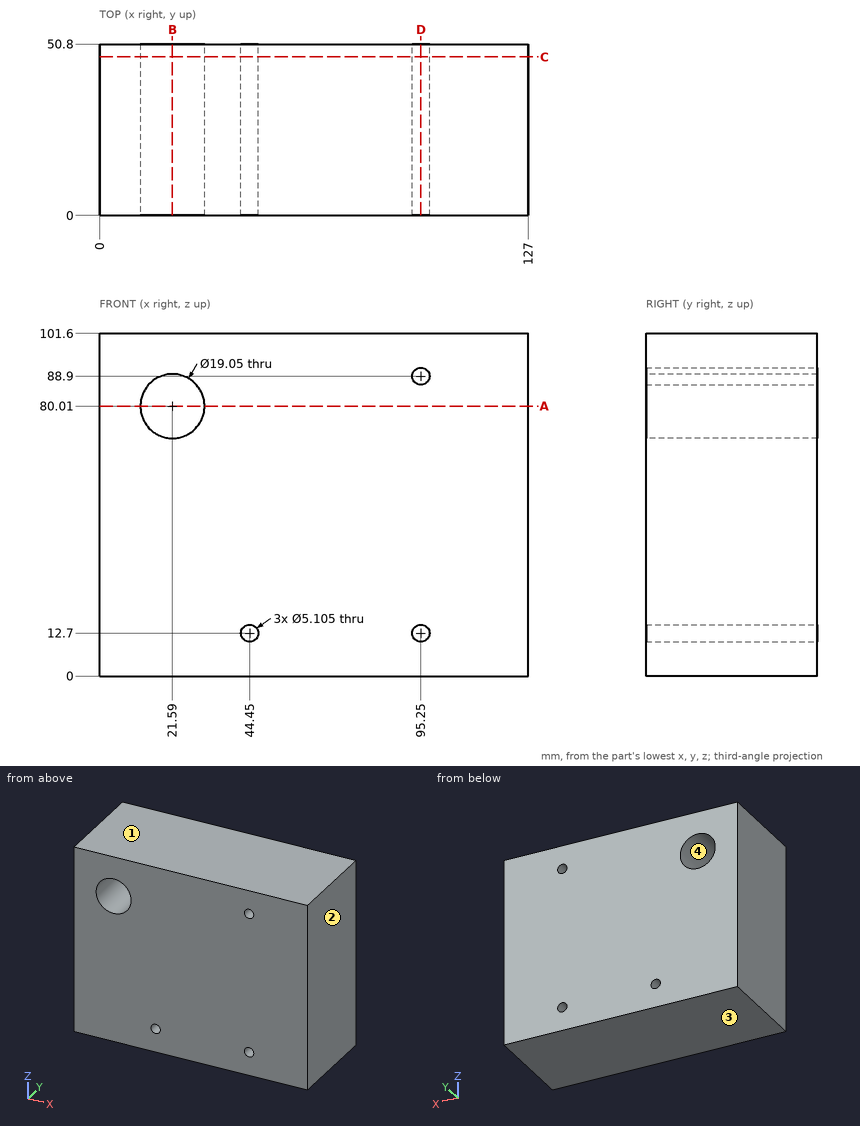
Study the drawing (mm; zero at the part's minimum x, y, z) and answer. Give positions to 0.01 mm unless a question says otherwise; leave off trailing zeros. Loops run counter-clockwise (first coordinate to the right, second up) from the corner with the lowest first, then second, coordinate; pieces in that order, holes last. Notation, with made-up numbers: M 23,79 L 28,79 A25 cw 28,108 Z; hole C 63,68 d6. An arc over 180 degrees is marked long. Answer as CSV lines item,"result".
Item 1: Straight lines are drawn through the part: line 1 along Z through (x, y) = (95.25, 40.5); line 2 along Z through (x, y) = (21.59, 14) (1 decimal); line 3 along X through (y, z) = (29, 80) (1 decimal). For each, find the intervals that lie inside material, in ascending order. Write a range as [from, to].
Values follow:
line 1,"z = [0, 10.15], [15.25, 86.35], [91.45, 101.6]"
line 2,"z = [0, 70.5], [89.5, 101.6]"
line 3,"x = [0, 12.1], [31.1, 127]"
Item 2: The part is cut by section C-C (y = 47). Give the number of separate pieces and of enclosed holes in the cut face, and give its area (3 significant figures).
Values follow:
separate pieces,"1"
enclosed holes,"4"
area,"12,600 mm^2"
Item 3: The part is cut by section A-A (z = 80.01). Give the vertices of the cut face in (x, y) (1 decimal).
Values follow:
outline,"M 0,0 L 12.1,0 L 12.1,50.8 L 0,50.8 Z; M 31.1,0 L 127,0 L 127,50.8 L 31.1,50.8 Z"
Item 4: The part is cut by section D-D (x = 95.25). Give the vertices of the cut face in (y, z), and give its area (3 significant figures).
Values follow:
outline,"M 0,0 L 50.8,0 L 50.8,10.15 L 0,10.15 Z; M 0,15.25 L 50.8,15.25 L 50.8,86.35 L 0,86.35 Z; M 0,91.45 L 50.8,91.45 L 50.8,101.6 L 0,101.6 Z"
area,"4,640 mm^2"
Item 5: The mould has two halves that part along Z. Classify the marked faces 1, 2, 3 and 4: released by +Z, released by -Z, zero draft, split by the parting line, or undercut.
Values follow:
face 1,"released by +Z"
face 2,"zero draft"
face 3,"released by -Z"
face 4,"undercut"
Item 6: Given pin 1 Ø15 at (x, z) = (21.59, 80.01) entering from -Y (3 decimals), flat-ended and moving along its own axis, determine where the tip first touches the part or whether it passes through.
Values follow:
pin 1,"passes through"
Item 7: The part is cut by section B-B (x = 21.59). Give the vertices of the cut face in (y, z) (1 decimal).
Values follow:
outline,"M 0,0 L 50.8,0 L 50.8,70.5 L 0,70.5 Z; M 0,89.5 L 50.8,89.5 L 50.8,101.6 L 0,101.6 Z"
